from build123d import *

# Parameters (mm, degrees)
F0_W     = 120
F0_H     = 90
F1_DEPTH = 20
F2_T     = -2.5


# Not quite as in the source:
# - a feature names something its author has since deleted; it is built from what else it names


with BuildPart() as f1:
    # F0 (on Top) → F1 (new body)
    with BuildSketch(Plane.XY):
        with Locations((0.2172155073, -0.1426615352)):
            Rectangle(F0_W, F0_H)
    extrude(amount=F1_DEPTH)

    # F2
    f2_openings = [f1.faces().sort_by_distance(p)[0] for p in [
        (0.217216, -0.142662, 20),
    ]]
    offset(amount=F2_T, openings=f2_openings)


solid = f1.part
Here's how the part is built. I have some questions about the finished solid (model axes, mm). A direction names the side the tool comes from. Round coordinates to 2 decimals unless told otherwise and drop trailing zeros. Loops run counter-clockwise (first coordinate to the right, second up) from the corner with the lowest first, then second, coordinate; pieces in that order, holes last. Notation, with made-up numbers: (63.25, 21) - (83.25, 21) arc R22 ccw to (83.25, 34) - close; hole circle Ø11 at (56.5, 37). An arc over 180 degrees is marked (long way). One line per question, with ' | ' between items. Start each with the question number.
Q1. I want a section at C-C (y = 2). Write out the boundary of the cut face in (x, z), then the cut area to 4 significant figures.
Q2. We'd pull the mould along X, two halves only. Please class faces 1 (the flat face through (60.217, -1, 10)), 2 (the flat face through (-1, 0, 0)), 3 (the flat face through (-59.783, -1, 10)), 4 (the flat face through (-1, 0, 2.5)): +X half, -X half, draft (parallel to the pull), parting line (faces both ways), or undercut.
Q3. I want a section at B-B (x = -17). Write out the boundary of the cut face in (y, z).
Q4. For faces 5 (the flat face through (-57.283, -1, 11)), 6 (the flat face through (-1, -45.143, 10)), which set-ups out of +Z, -Z, +X, -X, +Y, -Y let a thin tool reach every point of the face, with its end or its side?
Q5. Please list where these lines run through material, in increasing order: line 1 (Y direction, x = -46, z = 6.25); line 2 (X direction, y = 18.5, z = 19.25); line 3 (Z direction, x = 36, y = -20.5). Write a range as [from, to].
Q6. Will these pins go through, and if not, where does the flat tip stop? pin 1 (6 mm diameter, centred on x = 20, y = -30, fed in from +Z); pin 2 (1 mm diameter, centred on x = 22.5, y = -17, fed in from -Z).
Q7. I want a section at A-A (z = 6.25). Write out the boundary of the cut face in (x, y).
Response values:
1) outline: (-59.78, 0) - (60.22, 0) - (60.22, 20) - (57.72, 20) - (57.72, 2.5) - (-57.28, 2.5) - (-57.28, 20) - (-59.78, 20) - close | area: 387.5 mm²
2) face 1: +X half | face 2: draft | face 3: -X half | face 4: undercut
3) outline: (-45.14, 0) - (44.86, 0) - (44.86, 20) - (42.36, 20) - (42.36, 2.5) - (-42.64, 2.5) - (-42.64, 20) - (-45.14, 20) - close
4) face 5: +Z | face 6: +Z, -Z, +X, -X, -Y
5) line 1: y = [-45.14, -42.64], [42.36, 44.86] | line 2: x = [-59.78, -57.28], [57.72, 60.22] | line 3: z = [0, 2.5]
6) pin 1: stops at z = 2.5 | pin 2: stops at z = 0
7) outline: (-59.78, -45.14) - (60.22, -45.14) - (60.22, 44.86) - (-59.78, 44.86) - close; hole (-57.28, -42.64) - (57.72, -42.64) - (57.72, 42.36) - (-57.28, 42.36) - close
